from build123d import *

# Parameters (mm, degrees)
SKETCH_1_R      = 4
EXTRUDE_1_DEPTH = 20
SKETCH_2_R      = 6
EXTRUDE_2_DEPTH = 8
EXTRUDE_START   = 56
SKETCH_3_R      = 4
EXTRUDE_5_DEPTH = 56
FILLET_1_R      = 0.5
FILLET_2_R      = 0.5


with BuildPart() as part:
    # 草图1 → 凸台-拉伸1 (new body)
    with BuildSketch(Plane.XY):
        Circle(SKETCH_1_R)
    extrude(amount=EXTRUDE_1_DEPTH)

    # 草图2 → 凸台-拉伸2 (add)
    with BuildSketch(Plane.XY):
        Circle(SKETCH_2_R)
    extrude(amount=-EXTRUDE_2_DEPTH)

    # 草图3 → 凸台-拉伸5 (add)
    with BuildSketch(Plane(origin=(0, 0, -8), x_dir=(-1, 0, 0), z_dir=(0, 0, -1)).offset(EXTRUDE_START)):
        with Locations(Location((0, 0, 0), (0, 0, 180))):
            Circle(SKETCH_3_R)
    extrude(amount=-EXTRUDE_5_DEPTH)

    # 圆角1
    fillet_1_edges = [part.edges().sort_by_distance(p)[0] for p in [
        (-4, 0, 20),
    ]]
    fillet(fillet_1_edges, radius=FILLET_1_R)

    # 圆角2
    fillet_2_edges = [part.edges().sort_by_distance(p)[0] for p in [
        (-4, 0, -64),
        (-6, 0, 0),
        (-6, 0, -8),
    ]]
    fillet(fillet_2_edges, radius=FILLET_2_R)


solid = part.part
Geometry check sheet. Reference: the model listing, model coordinates, mm. A direction names the side the tool comes from. Give positions to 0.01 mm unless a question says otherwise; leave off trailing zeros. Loops run counter-clockwise (first coordinate to the right, second up) from the corner with the lowest first, then second, coordinate; pieces in that order, holes last. Notation, with made-up numbers: M 38,17.5 L 61,17.5 A23 ccw 61,53.5 Z; hole C 67,-6.75 d1. An arc over 180 degrees is marked long. Answer as a JSON object with one key per item and string values. Group by question number.
Item 1: Material ranges on L1, parallel to Z at x = -5.5, y = -0.25; L2, parallel to Y at x = 0, z = -29.5; L3, parallel to Z at x = -3.75, y = 0.5, recorded low to high.
Item 2: Sectioned sample at C-C on z = 12.5. Record the boundary of the cut face in (x, y), plus the area to 3 significant figures.
Item 3: Sectioned sample at A-A on x = 0. Record the boundary of the cut face in (y, z), plus the area to 3 significant figures.
Item 4: Access from +Z, -Z, +X, -X, +Y, -Y to the whole of each face (thin tool, end or side, straight path). Record for faces 1 (the cylindrical face through (-0.867, -3.905, 9.614)), 2 (the flat face through (-4, -2, -8)), 3 (the flat face through (0, 0, -64)).
Item 5: Gauge pin test, flat ends, axial feed: pin 1 (4 mm diameter, centred on x = 3, z = -14, fed in from +Y); pin 2 (1 mm diameter, centred on x = 4.5, y = 3, fed in from -Z); pin 3 (1.5 mm diameter, centred on x = 3, z = -36, fed in from -Y). Record the tip position at first contact, or that the pin passes through.
Findings below:
{
 "1": {"L1": "-8 to 0", "L2": "-4 to 4", "L3": "-63.91 to 19.91"},
 "2": {"outline": "C 0,0 d8", "area": "50.3 mm2"},
 "3": {"outline": "M -6,-7.5 A0.5 ccw -5.5,-8 L -4,-8 L -4,-63.5 A0.5 ccw -3.5,-64 L 3.5,-64 A0.5 ccw 4,-63.5 L 4,-8 L 5.5,-8 A0.5 ccw 6,-7.5 L 6,-0.5 A0.5 ccw 5.5,0 L 4,0 L 4,19.5 A0.5 ccw 3.5,20 L -3.5,20 A0.5 ccw -4,19.5 L -4,0 L -5.5,0 A0.5 ccw -6,-0.5 Z", "area": "704 mm2"},
 "4": {"face 1": "+Z", "face 2": "-Z", "face 3": "-Z, +X, -X, +Y, -Y"},
 "5": {"pin 1": "y = 3.87", "pin 2": "z = -8", "pin 3": "y = -3.31"}
}
